```python
from build123d import *

# Parameters (mm, degrees)
RESSALTO_EXTRUS_O2_DEPTH = 1.9
RESSALTO_EXTRUS_O3_DEPTH = 1.5
CORTE_EXTRUS_O1_DEPTH    = 100
ESBO_O5_W                = 0.8
ESBO_O5_H                = 6
RESSALTO_EXTRUS_O4_DEPTH = 1.5
CORTE_EXTRUS_O2_DEPTH    = 100
CORTE_EXTRUS_O3_DEPTH    = 1000


with BuildPart() as part:
    # Esboço1 → Ressalto-extrusão2 (new body)
    with BuildSketch(Plane.XY):
        with BuildLine():
            Line((-23.801253488, -0.31815777), (-23.801253488, -28.31815777))
            ThreePointArc((-23.801253488, -28.31815777), (-23.50836027, -29.025264551), (-22.801253488, -29.31815777))
            Line((-22.801253488, -29.31815777), (-16.801253488, -29.31815777))
            Line((-16.801253488, -29.31815777), (-16.801253488, -41.81815777))
            ThreePointArc((-16.801253488, -41.81815777), (-16.50836027, -42.525264551), (-15.801253488, -42.81815777))
            Line((-15.801253488, -42.81815777), (18.198746512, -42.81815777))
            ThreePointArc((18.198746512, -42.81815777), (18.905853293, -42.525264551), (19.198746512, -41.81815777))
            Line((19.198746512, -41.81815777), (19.198746512, 13.18184223))
            ThreePointArc((19.198746512, 13.18184223), (18.905853293, 13.888949011), (18.198746512, 14.18184223))
            Line((18.198746512, 14.18184223), (-15.801253488, 14.18184223))
            ThreePointArc((-15.801253488, 14.18184223), (-16.50836027, 13.888949011), (-16.801253488, 13.18184223))
            Line((-16.801253488, 13.18184223), (-16.801253488, 0.68184223))
            Line((-16.801253488, 0.68184223), (-22.801253488, 0.68184223))
            ThreePointArc((-22.801253488, 0.68184223), (-23.50836027, 0.388949011), (-23.801253488, -0.31815777))
        make_face()
    extrude(amount=RESSALTO_EXTRUS_O2_DEPTH)

    # Esboço3 → Ressalto-extrusão3 (add, symmetric)
    with BuildSketch(Plane.ZY.offset(16.801253488)):
        Polygon((1.9, -35.56815777), (1.9, -34.05815777), (3.5, -34.05815777), (3.5, -38.05815777), (1.9, -38.05815777), align=None)
        Polygon((1.9, 6.93184223), (1.9, 9.42184223), (3.5, 9.42184223), (3.5, 5.42184223), (1.9, 5.42184223), align=None)
    extrude(amount=RESSALTO_EXTRUS_O3_DEPTH, both=True)

    # Esboço4 → Corte-extrusão1 (cut)
    with BuildSketch(Plane(origin=(0, 0.68184223, 0), x_dir=(1, 0, 0), z_dir=(0, 1, 0))):
        Polygon((-23.801253488, 0), (-19.801253488, -1.9), (-23.801253488, -1.9), align=None)
    extrude(amount=-CORTE_EXTRUS_O1_DEPTH, mode=Mode.SUBTRACT)

    # Esboço5 → Ressalto-extrusão4 (add, symmetric)
    with BuildSketch(Plane(origin=(19.198746512, 0, 0), x_dir=(0, 0, -1), z_dir=(1, 0, 0))):
        with Locations((-2.3, -14.390539287)):
            Rectangle(ESBO_O5_W, ESBO_O5_H)
    extrude(amount=RESSALTO_EXTRUS_O4_DEPTH, both=True)

    # Esboço6 → Corte-extrusão2 (cut)
    with BuildSketch(Plane(origin=(0, -17.390539287, 0), x_dir=(-1, 0, 0), z_dir=(0, -1, 0))):
        Polygon((-20.698746512, -1.9), (-17.698746512, -2.7), (-20.698746512, -2.7), align=None)
    extrude(amount=-CORTE_EXTRUS_O2_DEPTH, mode=Mode.SUBTRACT)

    # Esboço7 → Corte-extrusão3 (cut)
    with BuildSketch(Plane(origin=(0, 9.42184223, 0), x_dir=(1, 0, 0), z_dir=(0, 1, 0))):
        Polygon((-15.301253488, -1.9), (-17.601253488, -3.5), (-15.301253488, -3.5), align=None)
    extrude(amount=-CORTE_EXTRUS_O3_DEPTH, mode=Mode.SUBTRACT)


solid = part.part
```
Model file for the job. Use its own axes, mm. A direction names the side the tool comes from. Give positions to 0.01 mm unless a question says otherwise; leave off trailing zeros. Order: outer loops, then holes, each group sorted by start corner. A loop starts at its lowest first (then second) coordinate and runs counter-clockwise, first axis right, second up.
1) Saw through at B-B, the plane z = 1.3. Write the cut outline in (x, y), then the cut area to 3 significant figures.
2) Saw through at C-C, the plane x = 6. Write the cut outline in (y, z).
3) 3-axis set-ups, long thin cutter, end or side, ignore diameter. For faces 4 (the flat face through (-18, -36, 1.9)), 5 (the flat face through (-16.801, 7, 1)), 6 (the flat face through (-19, -29.318, 1)): which of +Z, -Z, +X, -X, +Y, -Y reach the whole face in a straight line?
4) Mould opens along Y. For faces 1 (the flat face through (20, -14, 1.9)), 2 (the flat face through (-17.2, 9.422, 2.5)), 3 (the flat face through (-17.1, -34.058, 2.5)) say: +Y half, -Y half, draft (parallel to the pull), parting line (faces both ways), or undercut.
5) Saw through at D-D, the plane y = -15.5. Write the cut outline in (x, z), then the cut area to 3 significant figures.
6) Saw through at A-A, the plane y = 7. Write the cut outline in (x, z).
7) Wall check: probe 1 along Z at (x, y) = (18.5, 5.5); probe 2 along X at (y, z) = (12, 0.7); probe 3 along Y at (x, z) = (-18, 0.9). Give the ranges that are in metal, low to high.
8) Pin check, flat tips, straight feed: pin 1 (2 mm diameter, centred on x = 6.5, y = -34.5, fed in from +Z); pin 2 (2 mm diameter, centred on x = -19, z = 1, fed in from -Y); pin 3 (1.8 mm diameter, centred on x = -17, z = 2.5, fed in from -Y); pin 4 (0.5 mm diameter, centred on x = -16, z = 3, fed in from -Y). Stop position of each tip, or through.
Computed:
1. outline: (-21.06, -29.32) - (-16.8, -29.32) - (-16.8, -41.82) arc R1 ccw to (-15.8, -42.82) - (18.2, -42.82) arc R1 ccw to (19.2, -41.82) - (19.2, 13.18) arc R1 ccw to (18.2, 14.18) - (-15.8, 14.18) arc R1 ccw to (-16.8, 13.18) - (-16.8, 0.68) - (-21.06, 0.68) - close
1. area: 2,180 mm2
2. outline: (-42.82, 0) - (14.18, 0) - (14.18, 1.9) - (-42.82, 1.9) - close
3. face 4: -Z, -X, -Y
3. face 5: -Z, -X, +Y
3. face 6: +Z, -Z, -X, -Y
4. face 1: draft
4. face 2: +Y half
4. face 3: undercut
5. outline: (-23.8, 0) - (19.2, 0) - (19.2, 1.9) - (20.7, 1.9) - (17.7, 2.7) - (17.7, 1.9) - (-19.8, 1.9) - close
5. area: 79.1 mm2
6. outline: (-18.3, 1.9) - (-16.8, 1.9) - (-16.8, 0) - (19.2, 0) - (19.2, 1.9) - (-15.3, 1.9) - (-17.6, 3.5) - (-18.3, 3.5) - close
7. probe 1: z = 0 to 1.9
7. probe 2: x = -16.8 to 19.2
7. probe 3: y = -29.32 to 0.68
8. pin 1: stops at z = 1.9
8. pin 2: stops at y = -29.32
8. pin 3: stops at y = -42.67
8. pin 4: passes through
